Check sheet for the modelled part. Datum: model origin and axes. Units: mm. Coordinates: 2 decimals unless noted, no trailing zeros. Loops run counter-clockwise (first coordinate to the right, second up) from the corner with the lowest first, then second, coordinate; pieces in that order, holes last. Notation, with made-up numbers: (59, -4) -> (112, -4) arc R16 ccw to (112, 5) -> close; hole circle Ø8 at (54.25, 1). An arc over 180 degrees is marked (long way). Use one line per item in the form item = value.
from build123d import *

# Parameters (mm, degrees)
SKETCH_1_R          = 30
SKETCH_1_R_2        = 6
EXTRUDE_1_DEPTH     = 5
SKETCH_2_R          = 1.85
SKETCH_2_R_2        = 1.6
CUT_EXTRUDE_1_DEPTH = 10
SKETCH_3_R          = 2.6
CUT_EXTRUDE_2_DEPTH = 10
FILLET_1_R          = 200
FILLET_2_R          = 200
FILLET_3_R          = 200
FILLET_5_R          = 100
SKETCH_4_R          = 2.6
CUT_EXTRUDE_3_DEPTH = 10
SKETCH_5_RX         = 19.625454407
SKETCH_5_RY         = 13.166615993
CUT_EXTRUDE_4_DEPTH = 10
SKETCH_6_R          = 1.85
SKETCH_6_R_2        = 1.6
EXTRUDE_2_DEPTH     = 5.000001
SKETCH_7_R          = 1.85
CUT_EXTRUDE_5_DEPTH = 10


with BuildPart() as part:
    # 草图1 → 凸台-拉伸1 (new body)
    with BuildSketch(Plane.XY):
        with BuildLine():
            Line((-10.41889066, -59.088465181), (12.562442634, -78.372093471))
            Line((12.562442634, -78.372093471), (92.753346633, -173.939891406))
            Line((92.753346633, -173.939891406), (101.085014518, -196.830960785))
            ThreePointArc((101.085014518, -196.830960785), (126.7192698, -208.784410334), (138.672719349, -183.150155052))
            Line((138.672719349, -183.150155052), (125.846963974, -147.911681773))
            Line((125.846963974, -147.911681773), (80.5212086, -56.381557247))
            Line((80.5212086, -56.381557247), (60, 0))
            ThreePointArc((60, 0), (-38.567256581, 45.962666587), (-10.41889066, -59.088465181))
        make_face()
        Circle(SKETCH_1_R, mode=Mode.SUBTRACT)
        with Locations((119.878866933, -189.990557919)):
            Circle(SKETCH_1_R_2, mode=Mode.SUBTRACT)
    extrude(amount=EXTRUDE_1_DEPTH)

    # 草图2 → 切除-拉伸1 (cut)
    with BuildSketch(Plane.XY.offset(5)):
        with Locations((0, 44.5)):
            Circle(SKETCH_2_R)
        with Locations((31.466251763, 31.466251763)):
            Circle(SKETCH_2_R)
        with Locations((31.466251763, -31.466251763)):
            Circle(SKETCH_2_R)
        with Locations((0, -44.5)):
            Circle(SKETCH_2_R)
        with Locations((-31.466251763, -31.466251763)):
            Circle(SKETCH_2_R)
        with Locations((-31.466251763, 31.466251763)):
            Circle(SKETCH_2_R)
        with Locations((42.5, 0)):
            Circle(SKETCH_2_R_2)
        with Locations((-42.5, 0)):
            Circle(SKETCH_2_R)
    extrude(amount=-CUT_EXTRUDE_1_DEPTH, mode=Mode.SUBTRACT)

    # 草图3 → 切除-拉伸2 (cut)
    with BuildSketch(Plane.XY.offset(5)):
        with Locations((21.04758878, 50.813374288)):
            Circle(SKETCH_3_R)
        with Locations((50.813374288, 21.04758878)):
            Circle(SKETCH_3_R)
        with Locations((50.813374288, -21.04758878)):
            Circle(SKETCH_3_R)
        with Locations((21.04758878, -50.813374288)):
            Circle(SKETCH_3_R)
        with Locations((-21.04758878, -50.813374288)):
            Circle(SKETCH_3_R)
        with Locations((-50.813374288, -21.04758878)):
            Circle(SKETCH_3_R)
        with Locations((-50.813374288, 21.04758878)):
            Circle(SKETCH_3_R)
        with Locations((-21.04758878, 50.813374288)):
            Circle(SKETCH_3_R)
    extrude(amount=-CUT_EXTRUDE_2_DEPTH, mode=Mode.SUBTRACT)

    # 圆角1
    fillet_1_edges = [part.edges().sort_by_distance(p)[0] for p in [
        (125.846963974, -147.911681773, 2.5),
    ]]
    fillet(fillet_1_edges, radius=FILLET_1_R)

    # 圆角2
    fillet_2_edges = [part.edges().sort_by_distance(p)[0] for p in [
        (92.753346633, -173.939891406, 2.5),
    ]]
    fillet(fillet_2_edges, radius=FILLET_2_R)

    # 圆角3
    fillet_3_edges = [part.edges().sort_by_distance(p)[0] for p in [
        (12.562442634, -78.372093471, 2.5),
    ]]
    fillet(fillet_3_edges, radius=FILLET_3_R)

    # 圆角5
    fillet_5_edges = [part.edges().sort_by_distance(p)[0] for p in [
        (80.5212086, -56.381557247, 2.5),
        (60, 0, 2.5),
        (-10.41889066, -59.088465181, 2.5),
    ]]
    fillet(fillet_5_edges, radius=FILLET_5_R)

    # 草图4 → 切除-拉伸3 (cut)
    with BuildSketch(Plane.XY.offset(5)):
        with Locations((31.915052067, -63.622822556)):
            Circle(SKETCH_4_R)
        with Locations((51.725449506, -86.151651937)):
            Circle(SKETCH_4_R)
        with Locations((71.009077797, -109.132985231)):
            Circle(SKETCH_4_R)
        with Locations((90.292706088, -132.114318524)):
            Circle(SKETCH_4_R)
    extrude(amount=-CUT_EXTRUDE_3_DEPTH, mode=Mode.SUBTRACT)

    # 草图5 → 切除-拉伸4 (cut)
    with BuildSketch(Plane.XY.offset(5)):
        with Locations(Location((133.018329516, -157.967583367), (0, 0, -3.070599188))):
            Ellipse(SKETCH_5_RX, SKETCH_5_RY)
    extrude(amount=-CUT_EXTRUDE_4_DEPTH, mode=Mode.SUBTRACT)

    # 草图6 → 凸台-拉伸2 (add, through all)
    with BuildSketch(Plane.XY.offset(5)):
        with Locations((-44.5, 0)):
            Circle(SKETCH_6_R)
        with Locations((-42.5, 0)):
            Circle(SKETCH_6_R)
        with Locations((-44.5, 0)):
            Circle(SKETCH_6_R)
        with Locations((-42.5, 0)):
            Circle(SKETCH_6_R)
        with Locations((42.5, 0)):
            Circle(SKETCH_6_R_2)
        with Locations((44.5, 0)):
            Circle(SKETCH_6_R)
        with Locations((44.5, 0)):
            Circle(SKETCH_6_R)
        with Locations((42.5, 0)):
            Circle(SKETCH_6_R_2)
    extrude(amount=-EXTRUDE_2_DEPTH)

    # 草图7 → 切除-拉伸5 (cut)
    with BuildSketch(Plane.XY.offset(5)):
        with Locations((-44.5, 0)):
            Circle(SKETCH_7_R)
        with Locations((44.5, 0)):
            Circle(SKETCH_7_R)
    extrude(amount=-CUT_EXTRUDE_5_DEPTH, mode=Mode.SUBTRACT)


solid = part.part
(1) Section check A-A, the plane z = 4. Give the number of separate pieces and of enclosed holes in the cut face, plus the area to 3 significant figures.
Established:
separate_pieces = 1
enclosed_holes = 22
area = 18,000 mm²
(2) Section check B-B, the plane y = -38. Record the boundary of the cut face in (x, z).
Established:
outline = (-46.43, 0) -> (73.83, 0) -> (73.83, 5) -> (-46.43, 5) -> close
(3) Mould release check, pull along Y, two halves, no side actions. Record for faces 1 (the cylindrical face through (-35.435, 48.419, 2.465)), 2 (the cylindrical face through (48.75, 19.466, 2.535)), 3 (the cylindrical face through (16.89, -83.954, 2.535)): +Y half, -Y half, draft (parallel to the pull), parting line (faces both ways), or undercut.
Established:
face_1 = parting line
face_2 = undercut
face_3 = -Y half
(4) Scan lines: line 1 along Y through (x, z) = (52, 3.6); line 2 along Y through (x, z) = (50, 1.9); line 3 along Y through (x, z) = (-44.5, 3.5). Record each from-to range of solid material in increasing order.
Established:
line_1 = -125.37 to -88.74, -83.57 to -23.36, -18.73 to 18.73, 23.36 to 29.93
line_2 = -122.99 to -88.1, -84.21 to -23.52, -18.58 to 18.58, 23.52 to 33.17
line_3 = -40.25 to -1.85, 1.85 to 40.25
(5) Go/stop test with flat-tipped pins: P1, Ø2, axis at x = 31.47, y = 31.47, coming from the -Z side; P2, Ø2, axis at x = 115, z = 1, coming from the -Y side. Record where each tip stops, or that it passes through.
Established:
P1 = through
P2 = -209.61
